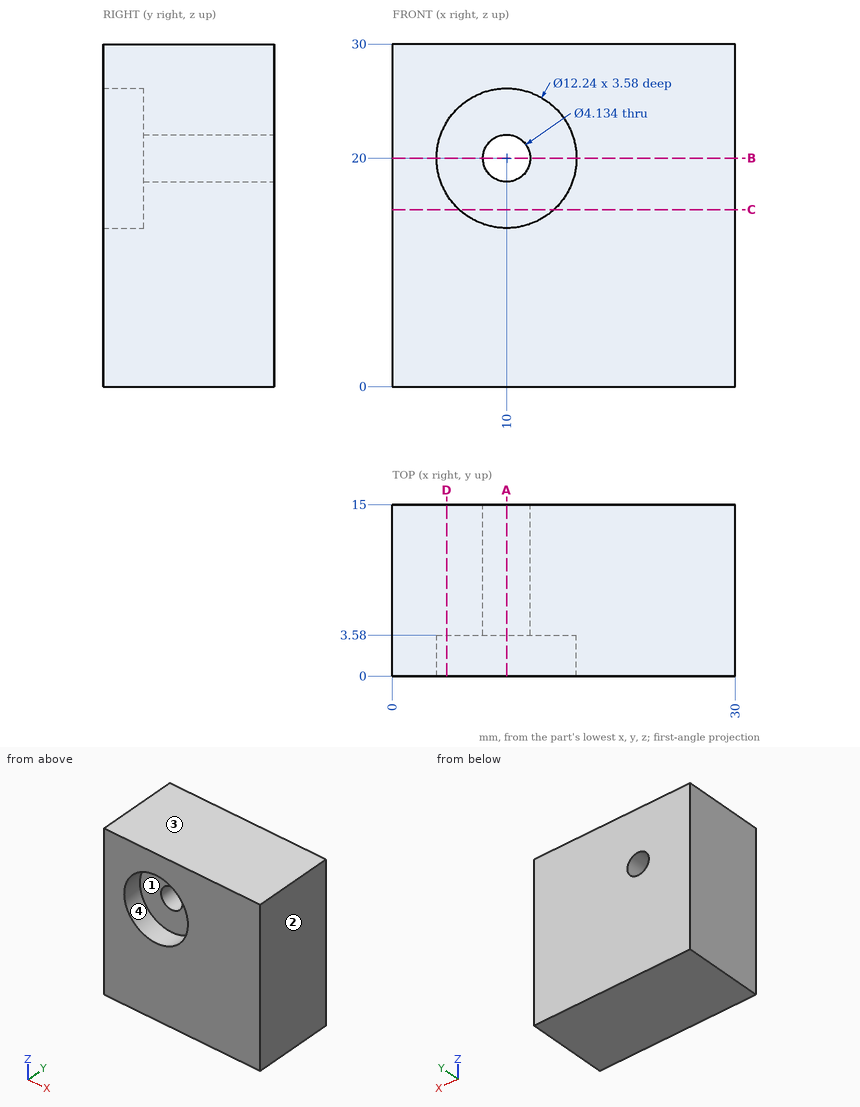
Study the drawing (mm; zero at the part's minimum x, y, z) and answer. Coordinates: 2 decimals unless noted, no trailing zeros. Order: outer loops, then holes, each group sorted by start corner. A loop starts at its lowest first (then second) coordinate and runs counter-clockwise, first axis right, second up. Notation, with made-up numbers: M -34,-8.75 L 7,-8.75 A16 ccw 7,22.25 Z; hole C -18,84 d7. An arc over 180 degrees is marked long. Use CSV: the item, a comma, the result in double quotes.
Q1. Section A-A (x = 10) is taken. Determine the outline of the cut face in (y, z).
Here are the results:
outline,"M 0,0 L 15,0 L 15,17.93 L 3.58,17.93 L 3.58,13.88 L 0,13.88 Z; M 0,26.12 L 3.58,26.12 L 3.58,22.07 L 15,22.07 L 15,30 L 0,30 Z"
Q2. Section D-D (x = 4.75) is taken. Determine the outline of the cut face in (y, z), then the cut area to 3 significant figures.
Here are the results:
outline,"M 0,0 L 15,0 L 15,30 L 0,30 L 0,23.15 L 3.58,23.15 L 3.58,16.85 L 0,16.85 Z"
area,"427 mm2"
Q3. Section C-C (z = 15.5) is taken. Determine the outline of the cut face in (x, y), then the cut area to 3 significant figures.
Here are the results:
outline,"M 0,0 L 5.85,0 L 5.85,3.58 L 14.15,3.58 L 14.15,0 L 30,0 L 30,15 L 0,15 Z"
area,"420 mm2"
Q4. Section B-B (z = 20) is taken. Determine the outline of the cut face in (x, y).
Here are the results:
outline,"M 0,0 L 3.88,0 L 3.88,3.58 L 7.93,3.58 L 7.93,15 L 0,15 Z; M 12.07,3.58 L 16.12,3.58 L 16.12,0 L 30,0 L 30,15 L 12.07,15 Z"
Q5. Determine the mould class of the marked faces 1, 2, 3 and 4 for opening direction Z: pulls with the +Z half, pulls with the -Z half, needs draft (parallel to the pull), parting line crosses it, or undercut.
Here are the results:
face 1,"undercut"
face 2,"needs draft"
face 3,"pulls with the +Z half"
face 4,"undercut"
Q6. Straight lines are drawn through the part: L1, parallel to X at y = 7.75, z = 20; L2, parallel to Z at x = 10, y = 2.05; L3, parallel to X at y = 2.35, z = 20. For each, find the intervals that lie inside material, in ascending order.
Here are the results:
L1,"0 to 7.93, 12.07 to 30"
L2,"0 to 13.88, 26.12 to 30"
L3,"0 to 3.88, 16.12 to 30"
